The listing builds one solid part. Answer for the finished solid, in the listing's coordinates (mm). A direction names the side the tool comes from. Round coordinates to 2 decimals unless told otherwise and drop trailing zeros. Order: outer loops, then holes, each group sorted by start corner. A loop starts at its lowest first (then second) coordinate and runs counter-clockwise, first axis right, second up. Notation, with made-up numbers: (31, 85) -> (68, 85) arc R20 ccw to (68, 105) -> close; hole circle Ø3 at (83.5, 7.25). An arc over 180 degrees is marked (long way). Return JSON: item names as keys, results as strings. Group by question number.
(1) The part is cut by section C-C (z = 0.25). Determine the outline of the cut face in (x, y).
(2) The part is cut by section B-B (x = 0). Determine the outline of the cut face in (y, z).
(3) The part is cut by section D-D (y = 3). Determine the outline of the cut face in (x, z), plus the area to 3 significant figures.
(4) Each of these flat-tipped pins is pushed along its axis until it touches: pin 1 (0.6 mm diameter, centred on x = 3.5, z = -1, fed in from -Y); pin 2 (4 mm diameter, centred on x = -0.5, z = -1, fed in from -Y); pin 3 (2.5 mm diameter, centred on x = 0.5, y = 4, fed in from +Z); pin 4 (1.2 mm diameter, centred on y = 5, z = 2.5, fed in from +X). Where does it stop, or does it pass through?
(5) Which of the six approach directions +Z, -Z, +X, -X, +Y, -Y give full straight-line access (tool end or side, diameter ignored) to faces 1 (the face through (0.925, -0.5, -3.4)), 2 (the face through (3.599, -0.507, -0.507)), 3 (the face through (0, 3, 4))?
(6) Consider line 1 (X direction, y = 5.25, z = 0); line 2 (X direction, y = 3.75, z = -2); line 3 (X direction, y = 2.5, z = -0.5). Determine where each line is inside the solid, lowest interval first. Write a range as [from, to].
(7) Determine the mould class of faces 4 (the face through (-4, 3, 2)), 5 (the face through (4, 3.8, 1.5)), 6 (the face through (-3, 0, 1)), 7 (the face through (6.405, 1.465, -3.381)) for opening direction X: +X half, -X half, draft (parallel to the pull), parting line (faces both ways), or undercut.
(8) The part is cut by section A-A (y = -0.5). Determine the outline of the cut face in (x, z).
from build123d import *

# Parameters (mm, degrees)
SKETCH1_R           = 3
BOSS_EXTRUDE1_DEPTH = 7
BOSS_EXTRUDE2_START = 1
BOSS_EXTRUDE2_DEPTH = 1
BOSS_EXTRUDE6_DEPTH = 5


with BuildPart() as part:
    # Sketch1 → Boss-Extrude1 (new body)
    with BuildSketch(Plane(origin=(0, 0, 0), x_dir=(1, 0, 0), z_dir=(0, 1, 0))):
        with BuildLine():
            Line((4, 0), (4, -4))
            Line((4, -4), (-4, -4))
            Line((-4, -4), (-4, 0))
            ThreePointArc((-4, 0), (0, 4), (4, 0))
        make_face()
        with Locations(Location((0, 0, 0), (0, 0, 90))):
            Circle(SKETCH1_R, mode=Mode.SUBTRACT)
    extrude(amount=BOSS_EXTRUDE1_DEPTH)

    # Sketch4 → Boss-Extrude2 (add)
    with BuildSketch(Plane.XZ.offset(BOSS_EXTRUDE2_START)):
        with BuildLine():
            Line((4, 0), (4, 4))
            Line((4, 4), (0.924622027, 4))
            Line((0.924622027, 4), (0.924622027, 2.853957622))
            ThreePointArc((0.924622027, 2.853957622), (2.426300278, 1.764388551), (3, 0))
            ThreePointArc((3, 0), (2.426300278, -1.764388551), (0.924622027, -2.853957622))
            Line((0.924622027, -2.853957622), (0.924622027, -3.891667266))
            Line((0.924622027, -3.891667266), (4, 0))
        make_face()
    extrude(amount=-BOSS_EXTRUDE2_DEPTH)

    # Sketch6 → Boss-Extrude6 (add)
    with BuildSketch(Plane.XZ.offset(1)):
        with BuildLine():
            Line((3.209082629, -1.000848439), (2.532928766, -1.856472001))
            ThreePointArc((2.532928766, -1.856472001), (6.465725292, -3.364130595), (9, 0))
            Line((9, 0), (9, 4.051493621))
            Line((9, 4.051493621), (4, 4))
            Line((4, 4), (4, 2))
            ThreePointArc((4, 2), (6.618033989, 2.236067977), (8, 0))
            ThreePointArc((8, 0), (6.011227235, -2.447171166), (3.209082629, -1.000848439))
        make_face()
    extrude(amount=-BOSS_EXTRUDE6_DEPTH)


solid = part.part
Answer below:
{
 "1": {"outline": "(-4, 0) -> (-2.99, 0) -> (-2.99, 7) -> (-4, 7) -> close; (2.99, -1) -> (4, -1) -> (4, 7) -> (2.99, 7) -> close; (7.99, -1) -> (9, -1) -> (9, 4) -> (7.99, 4) -> close"},
 "2": {"outline": "(0, -4) -> (7, -4) -> (7, -3) -> (0, -3) -> close; (0, 3) -> (7, 3) -> (7, 4) -> (0, 4) -> close"},
 "3": {"outline": "(-4, 0) arc R4 ccw to (3.09, -2.54) arc R3.5 ccw to (9, 0) -> (9, 4.05) -> (4, 4) -> (-4, 4) -> close; hole circle Ø6 at (0, 0); hole (3.64, -1.67) arc R2.5 ccw (long way) to (4, 2) -> (4, 0) arc R4 cw to start", "area": "47.6 mm²"},
 "4": {"pin 1": "stops at y = -1", "pin 2": "stops at y = 0", "pin 3": "stops at z = 4", "pin 4": "stops at x = 4"},
 "5": {"face 1": "+Z, -Z, -X, -Y", "face 2": "-Y", "face 3": "+Z, -X, +Y, -Y"},
 "6": {"line 1": "x = [-4, -3], [3, 4]", "line 2": "x = [-3.46, -2.24], [2.24, 4], [7, 8.37]", "line 3": "x = [-3.97, -2.96], [2.96, 3.97], [7.95, 8.96]"},
 "7": {"face 4": "-X half", "face 5": "undercut", "face 6": "draft", "face 7": "undercut"},
 "8": {"outline": "(0.92, -3.89) -> (2.53, -1.86) arc R3.5 ccw to (9, 0) -> (9, 4.05) -> (4, 4) -> (0.92, 4) -> (0.92, 2.85) arc R3 cw to (0.92, -2.85) -> close; hole (3.21, -1) arc R2.5 ccw (long way) to (4, 2) -> (4, 0) -> close"}
}
